The listing builds one solid part. Answer for the finished solid, in the listing's coordinates (mm). A direction names the side the tool comes from. Round coordinates to 2 decimals unless told otherwise and drop trailing zeros. Loops run counter-clockwise (first coordinate to the right, second up) from the corner with the lowest first, then second, coordinate; pieces in that order, holes last. Notation, with made-up numbers: M -29.5,-15.5 L 15.5,-15.5 A19 ccw 15.5,-3.5 Z; hole C -22,-27 d2. An arc over 180 degrees is marked long. Answer as a JSON object with one key per item and string values.
Autodesk Inventor part; units mm, degrees
ref_plane "YZ Plane" through (0, 0, 0) normal (1, 0, 0) x (0, 1, 0)
ref_plane "XZ Plane" through (0, 0, 0) normal (0, 1, 0) x (-1, 0, 0)
ref_plane "XY Plane" through (0, 0, 0) normal (0, 0, 1) x (1, 0, 0)
sketch "Sketch1" plane through (0, 0, 0) normal (0, 1, 0) x (-1, 0, 0)
  circle A0 centre (0, 0) radius 15
  dimension "d0" = 30
extrude "Extrusion1" add sketch "Sketch1" along normal blind 35
sketch "Sketch2" plane through (0, 0, 0) normal (0, -1, 0) x (1, 0, 0)
  circle A0 centre (0, 0) radius 10
  circle A1 centre (0, 0) radius 15
  dimension "d3" = 20
extrude "Extrusion2" cut sketch "Sketch2" against normal blind 5
sketch "Sketch3" plane through (0, 35, 0) normal (0, 1, 0) x (1, 0, 0)
  circle A0 centre (0, 0) radius 2.5
  dimension "d6" = 5
extrude "Extrusion3" add sketch "Sketch3" along normal blind 15
sketch "Sketch4" plane through (0, 50, 0) normal (0, 1, 0) x (1, 0, 0)
  circle A0 centre (0, 0) radius 2.5
  line L0 (-1.5, -3.5) -> (1.5, -3.5)
  line L1 (1.5, -3.5) -> (1.5, 3.5)
  line L2 (1.5, 3.5) -> (-1.5, 3.5)
  line L3 (-1.5, 3.5) -> (-1.5, -3.5)
  circle A1 centre (0, 0) radius 2.5
  line L4 (-1.5, -3.5) -> (1.5, 3.5) construction
  line L5 (1.5, -3.5) -> (-1.5, 3.5) construction
  point P0 (1.5, 2)
  point P1 (1.5, -2)
  dimension "d9" = 3
  dimension "d10" = 7
extrude "Extrusion4" cut sketch "Sketch4" against normal blind 10 contours A0 L1
properties part number "Motor"
Item 1: Which of the six approach directions +Z, -Z, +X, -X, +Y, -Y give full straight-line access (tool end or side, diameter ignored) to faces 1 (the face through (-2.5, 42.4, 0.1)), 2 (the face through (3, 5, -10)), 3 (the face through (2, 40, 0)), 4 (the face through (0, 0, 0)), 5 (the face through (-1, 50, 0))?
Values follow:
{"face 1": "+Y", "face 2": "-Y", "face 3": "+Z, -Z, +X, +Y", "face 4": "+Z, -Z, +X, -X, -Y", "face 5": "+Z, -Z, +X, -X, +Y"}
Item 2: The part is cut by section C-C (y = 18). Give the vertices of the cut face in (x, z).
Values follow:
{"outline": "C 0,0 d30"}
Item 3: The part is cut by section A-A (x = 0). Give the vertices of the cut face in (y, z).
Values follow:
{"outline": "M 0,-10 L 5,-10 L 5,-15 L 35,-15 L 35,-2.5 L 50,-2.5 L 50,2.5 L 35,2.5 L 35,15 L 5,15 L 5,10 L 0,10 Z"}
Item 4: Straight lines are drawn through the part: line 1 (Z direction, x = -0.5, y = 29.5); line 2 (Y direction, x = -12.5, z = -4.5); line 3 (Y direction, x = 1.5, z = 4.25). For each, find the intervals that lie inside material, in ascending order.
Values follow:
{"line 1": "-14.99 to 14.99", "line 2": "5 to 35", "line 3": "0 to 35"}
Item 5: The part is cut by section B-B (z = 0). Give the vertices of the cut face in (x, y).
Values follow:
{"outline": "M -15,5 L -10,5 L -10,0 L 10,0 L 10,5 L 15,5 L 15,35 L 2.5,35 L 2.5,40 L 1.5,40 L 1.5,50 L -2.5,50 L -2.5,35 L -15,35 Z"}
Item 6: Flat-ended cylindrical pins translate along their axes: P1, Ø6, axis at x = -1, z = 11.5, coming from the -Y side; P2, Ø3, axis at y = 13, z = 4, coming from the -X side; P3, Ø5, axis at x = -0.5, z = 10.5, coming from the +Y side; P4, Ø3, axis at y = 14.5, z = 5.5, coming from the +X side. Find the tip coordinate at first contact, or state that the pin passes through.
Values follow:
{"P1": "y = 0", "P2": "x = -14.79", "P3": "y = 35", "P4": "x = 14.46"}
Item 7: The part is cut by section D-D (x = -3.75). Give the vertices of the cut face in (y, z).
Values follow:
{"outline": "M 0,-9.27 L 5,-9.27 L 5,-14.52 L 35,-14.52 L 35,14.52 L 5,14.52 L 5,9.27 L 0,9.27 Z"}
